Check sheet for the modelled part. Datum: model origin and axes. Units: mm. A direction names the side the tool comes from. Round coordinates to 2 decimals unless told otherwise and drop trailing zeros. Order: outer loops, then holes, each group sorted by start corner. A loop starts at its lowest first (then second) coordinate and runs counter-clockwise, first axis right, second up. Notation, with made-up numbers: (33.5, 72.25) -> (40.5, 72.25) arc R18 cw to (40.5, 90.25) -> close; hole circle Ø10 at (40.5, 18.25). An arc over 180 degrees is marked (long way). Answer in a Markdown table with one row per item.
```python
from build123d import *

# Parameters (mm, degrees)
RESSALTO_EXTRUS_O1_DEPTH = 30
ESBO_O4_R                = 6
CORTE_EXTRUS_O1_DEPTH    = 4
ESBO_O5_R                = 5
CORTE_EXTRUS_O2_DEPTH    = 11
ESBO_O6_R                = 1.5
CORTE_EXTRUS_O3_DEPTH    = 54.749418602
ESBO_O7_R                = 2.5
CORTE_EXTRUS_O4_DEPTH    = 9
ESBO_O8_R                = 2
CORTE_EXTRUS_O5_DEPTH    = 11


with BuildPart() as part:
    # Esboço2 → Ressalto-extrusão1 (new body)
    with BuildSketch(Plane.XY):
        Polygon((0, 0), (0, -42), (15, -42), (15, -10), (10, -10), (10, 0), align=None)
    extrude(amount=RESSALTO_EXTRUS_O1_DEPTH)

    # Esboço4 → Corte-extrusão1 (cut)
    with BuildSketch(Plane(origin=(15, 0, 0), x_dir=(0, 0, -1), z_dir=(1, 0, 0))):
        with Locations((-15, -22)):
            Circle(ESBO_O4_R)
    extrude(amount=-CORTE_EXTRUS_O1_DEPTH, mode=Mode.SUBTRACT)

    # Esboço5 → Corte-extrusão2 (cut)
    with BuildSketch(Plane.ZY):
        with Locations(Location((15, -22, 0), (0, 0, 270))):
            Circle(ESBO_O5_R)
    extrude(amount=-CORTE_EXTRUS_O2_DEPTH, mode=Mode.SUBTRACT)

    # Esboço6 → Corte-extrusão3 (cut, through all)
    with BuildSketch(Plane.XY.offset(30)):
        with Locations((7.5, -17)):
            Circle(ESBO_O6_R)
    extrude(amount=-CORTE_EXTRUS_O3_DEPTH, mode=Mode.SUBTRACT)

    # Esboço7 → Corte-extrusão4 (cut)
    with BuildSketch(Plane.XZ.offset(42)):
        with Locations(Location((7.097716039, 24, 0), (0, 0, 270))):
            Circle(ESBO_O7_R)
        with Locations(Location((7.097716039, 6, 0), (0, 0, 270))):
            Circle(ESBO_O7_R)
    extrude(amount=-CORTE_EXTRUS_O4_DEPTH, mode=Mode.SUBTRACT)

    # Esboço8 → Corte-extrusão5 (cut)
    with BuildSketch(Plane.XZ.offset(42)):
        with Locations(Location((7.097716039, 24, 0), (0, 0, 270))):
            Circle(ESBO_O8_R)
        with Locations(Location((7.097716039, 6, 0), (0, 0, 270))):
            Circle(ESBO_O8_R)
    extrude(amount=-CORTE_EXTRUS_O5_DEPTH, mode=Mode.SUBTRACT)


solid = part.part
```
(1) Section check B-B on y = -22. Record the boundary of the cut face in (x, z).
Solutions:
| item | result |
|---|---|
| outline | (0, 0) -> (15, 0) -> (15, 9) -> (11, 9) -> (11, 10) -> (0, 10) -> close; (0, 20) -> (11, 20) -> (11, 21) -> (15, 21) -> (15, 30) -> (0, 30) -> close |
(2) Section check D-D on x = 2.5. Record the boundary of the cut face in (y, z).
Solutions:
| item | result |
|---|---|
| outline | (-42, 0) -> (0, 0) -> (0, 30) -> (-42, 30) -> close; hole circle Ø10 at (-22, 15) |
(3) Scan lines: probe 1 along Y at (x, z) = (3, 15); probe 2 along X at (y, z) = (-35, 24); probe 3 along Y at (x, z) = (7.5, 3.5). Record each from-to range of solid material in increasing order. Write a range as from..to.
Solutions:
| item | result |
|---|---|
| probe 1 | -42..-27, -17..0 |
| probe 2 | 0..4.6, 9.6..15 |
| probe 3 | -42..-18.5, -15.5..0 |
(4) Section check C-C on z = 17. Record the boundary of the cut face in (x, y), plus the area to 3 significant figures.
Solutions:
| item | result |
|---|---|
| outline | (0, -42) -> (15, -42) -> (15, -27.66) -> (11, -27.66) -> (11, -26.58) -> (0, -26.58) -> close; (0, -17.42) -> (6.06, -17.42) arc R1.5 cw (long way) to (8.94, -17.42) -> (11, -17.42) -> (11, -16.34) -> (15, -16.34) -> (15, -10) -> (10, -10) -> (10, 0) -> (0, 0) -> close |
| area | 429 mm^2 |
(5) Section check A-A on z = 24. Record the boundary of the cut face in (x, y), plus the area to 3 significant figures.
Solutions:
| item | result |
|---|---|
| outline | (0, -42) -> (4.6, -42) -> (4.6, -33) -> (5.1, -33) -> (5.1, -31) -> (9.1, -31) -> (9.1, -33) -> (9.6, -33) -> (9.6, -42) -> (15, -42) -> (15, -10) -> (10, -10) -> (10, 0) -> (0, 0) -> close; hole circle Ø3 at (7.5, -17) |
| area | 520 mm^2 |
(6) Tool access check on faces 1 (the cylindrical face through (5.6, -37.6, 26)), 2 (the flat face through (15, -30, 15)), 3 (the flat face through (0, -16, 15)), 4 (the cylindrical face through (13.028, -20.198, 9.277)), 5 (the flat face through (10, -5, 15)). Record the directions out of +Z, -Z, +X, -X, +Y, -Y that give a thin tool (end or side, any length) a straight path to the whole face; none if there is none.
Solutions:
| item | result |
|---|---|
| face 1 | -Y |
| face 2 | +Z, -Z, +X, +Y, -Y |
| face 3 | +Z, -Z, -X, +Y, -Y |
| face 4 | +X |
| face 5 | +Z, -Z, +X, +Y |
(7) Depth check by flat-ended pin: pin 1 Ø2.5 at (x, z) = (8, 5) entering from -Y; pin 2 Ø3 at (x, z) = (7.5, 5.5) entering from -Y; pin 3 Ø5 at (y, z) = (-6.5, 14) entering from +X; pin 4 Ø3 at (x, z) = (7.1, 6) entering from -Y. Enter the tip coordinate at first touch or a pass-through.
Solutions:
| item | result |
|---|---|
| pin 1 | y = -42 |
| pin 2 | y = -33 |
| pin 3 | x = 10 |
| pin 4 | y = -31 |
(8) Draft check along Y on faces 6 (the cylindrical face through (4.88, -37.56, 4.85)), 7 (the flat face through (7, -31, 24)), 8 (the flat face through (11, -18, 19)). Enter one of: pulls with the +Y half, pulls with the -Y half, needs draft (parallel to the pull), parting line crosses it, or undercut.
Solutions:
| item | result |
|---|---|
| face 6 | needs draft |
| face 7 | pulls with the -Y half |
| face 8 | undercut |
